Autodesk Inventor part; units mm, degrees
ref_plane "YZ Plane" through (0, 0, 0) normal (1, 0, 0) x (0, 1, 0)
ref_plane "XZ Plane" through (0, 0, 0) normal (0, 1, 0) x (-1, 0, 0)
ref_plane "XY Plane" through (0, 0, 0) normal (0, 0, 1) x (1, 0, 0)
sketch "Esboço1" plane through (0, 0, 0) normal (0, 0, 1) x (1, 0, 0)
  line L0 (15.7389, -119.5954) -> (21.8039, -119.5954)
  line L1 (21.8039, -119.5954) -> (21.8039, -45.5852)
  line L2 (10.4016, -45.5852) -> (10.4016, -32.1476)
  line L3 (20.3752, -32.1476) -> (20.3752, 0.0017)
  arc A0 (-20.7435, 0.0017) -> (15.7389, -119.5954) centre (201.4548, 2.419) ccw
  circle A1 centre (15.3884, -57.4534) radius 2.5
  line L4 (21.8039, -45.5852) -> (10.4016, -45.5852)
  line L5 (20.3752, -32.1476) -> (10.4016, -32.1476)
  line L6 (20.3752, 0.0017) -> (13.075, 0.0017)
  arc A2 (15.7389, 119.5989) -> (-20.7435, 0.0017) centre (201.4548, -2.4155) ccw
  line L7 (20.3752, 32.1511) -> (20.3752, 0.0017)
  circle A3 centre (15.3884, 57.4569) radius 2.5
  line L8 (10.4016, 45.5887) -> (10.4016, 32.1511)
  line L9 (15.7389, 119.5989) -> (21.8039, 119.5989)
  line L10 (21.8039, 45.5887) -> (10.4016, 45.5887)
  line L11 (20.3752, 32.1511) -> (10.4016, 32.1511)
  line L12 (21.8039, 45.5887) -> (21.8039, 119.5989)
  circle A4 centre (5.3884, -57.4534) radius 2.5
  circle A5 centre (5.3884, 57.4569) radius 2.5
  point P0 (0, 0)
  dimension "d0" = 5
  dimension "d6" = 10
  dimension "d13" = 10
extrude "Extrusão1" add sketch "Esboço1" along normal blind 1
properties part number "sensor2"
Could you check a few things on this model? Use its own coordinates, in mm. Coordinates: 2 decimals unless noted, no trailing zeros. Write each loop counter-clockwise with the first axis right and the second up, starting at its lowest first coordinate (ties: lowest second). Pieces come first, ordered by that corner, then holes. Notation, with made-up numbers: (-35, 56) - (-15, 56) arc R15 cw to (-15, 73) - close; hole circle Ø10 at (72, 71). An arc over 180 degrees is marked (long way). Write item = value, one per line.
1) Please list where these lines run through material, in increasing order: line 1 (Y direction, x = 19, z = 0.65); line 2 (X direction, y = -57.5, z = 0.75); line 3 (Y direction, x = 4, z = 0.5). Write a range as [from, to].
Result set:
line_1 = [-119.6, -45.59], [-32.15, 32.15], [45.59, 119.6]
line_2 = [-12.53, 2.89], [7.89, 12.89], [17.89, 21.8]
line_3 = [-99.51, -59.53], [-55.37, 55.38], [59.54, 99.51]
2) Suppose I cut it at C-C on x = -15.5. Please give me the cut outline in (y, z).
Result set:
outline = (-45.63, 0) - (45.63, 0) - (45.63, 1) - (-45.63, 1) - close
3) Suppose I cut it at B-B on y = -67. Please give me the cut outline in (x, z), plus the area to 3 significant figures.
Result set:
outline = (-9.64, 0) - (21.8, 0) - (21.8, 1) - (-9.64, 1) - close
area = 31.4 mm2
4) Suppose I cut it at A-A on z = 0.45. Please give me the cut outline in (x, y), plus the area to 3 significant figures.
Result set:
outline = (-20.74, 0) arc R222.21 ccw to (15.74, -119.6) - (21.8, -119.6) - (21.8, -45.59) - (10.4, -45.59) - (10.4, -32.15) - (20.38, -32.15) - (20.38, 32.15) - (10.4, 32.15) - (10.4, 45.59) - (21.8, 45.59) - (21.8, 119.6) - (15.74, 119.6) arc R222.21 ccw to start; hole circle Ø5 at (5.39, -57.45); hole circle Ø5 at (5.39, 57.46); hole circle Ø5 at (15.39, -57.45); hole circle Ø5 at (15.39, 57.46)
area = 6,840 mm2
5) We'd pull the mould along X, two halves only. Please class faces 1 (the cylindrical face through (4.85, 59.9, 0.49)), 2 (the cylindrical face through (14.85, 59.9, 0.49)), 3 (the cylindrical face through (-10.83, -63.26, 0.49)), 4 (the flat face through (5, 2, 1)): +X half, -X half, draft (parallel to the pull), parting line (faces both ways), or undercut.
Result set:
face_1 = undercut
face_2 = undercut
face_3 = -X half
face_4 = draft
6) Will this pin go through, and if not, where does the flat tip stop? pin 1 Ø5 at (x, y) = (-3.5, 83) entering from -Z.
Result set:
pin_1 = 0
